from build123d import *

# Parameters (mm, degrees)
F0_R     = 29.1968279335
F1_DEPTH = 46.8261539936
F2_W     = 38.307864219
F2_H     = 7.8112371266
F3_DEPTH = 36.9160473347
F4_R     = 15.8391842582
F5_DEPTH = 29.1978279335
F6_T     = -2.54


with BuildPart() as f1:
    # F0 (on Top) → F1 (new body)
    with BuildSketch(Plane.XY):
        Circle(F0_R)
    extrude(amount=F1_DEPTH)

    # F2 (on face) → F3 (join)
    with BuildSketch(Plane.XY.offset(46.8261539936)):
        with Locations((0, 3.9056185633)):
            Rectangle(F2_W, F2_H)
    extrude(amount=F3_DEPTH)

    # F4 (on face) → F5 (cut, through all)
    with BuildSketch(Plane.XZ):
        with Locations((0, 64.5071235189)):
            Circle(F4_R)
        with BuildLine():
            ThreePointArc((-19.1539321095, 65.2841776609), (0, 83.6768112679), (19.1539321095, 65.2841776609))
            Line((19.1539321095, 65.2841776609), (19.1539321095, 83.7422013283))
            Line((19.1539321095, 83.7422013283), (-19.1539321095, 83.7422013283))
            Line((-19.1539321095, 83.7422013283), (-19.1539321095, 65.2841776609))
        make_face()
    extrude(amount=-F5_DEPTH, mode=Mode.SUBTRACT)

    # F6
    f6_openings = [f1.faces().sort_by_distance(p)[0] for p in [
        (0, 0, 0),
    ]]
    offset(amount=F6_T, openings=f6_openings, kind=Kind.INTERSECTION)


solid = f1.part
Source: CAD feature listing. Evaluate the final solid. Frame: model axes, mm. A direction names the side the tool comes from. Round coordinates to 2 decimals unless told otherwise and drop trailing zeros. Loops run counter-clockwise (first coordinate to the right, second up) from the corner with the lowest first, then second, coordinate; pieces in that order, holes last. Notation, with made-up numbers: (-5, 3.5) -> (0, 3.5) arc R36 cw to (0, 40.5) -> close; hole circle Ø1 at (23, -21.75). An arc over 180 degrees is marked (long way). Answer as a JSON object with one key per item and string values. Group by question number.
Q1. Section query B-B (z = 71.5). Output: boundary loops of the cut face in (x, y).
Q2. Access query for faces 4 (the flat face through (19.154, 4, 56)), 5 (the cylindrical face through (-5.779, -26.023, 21.833)), 6 (the flat face through (-19.154, 4, 56)). Directions: +Z, -Z, +X, -X, +Y, -Y. A direction counts if a zero-diameter tool reaches every point of the face in a straight line with its end or side. Return the directions, or none.
Q3. Mould query, pull axis X, two halves, no side actions, for faces 1 (the cylindrical face through (-0.411, 3.851, 83.672)), 2 (the flat face through (-2.927, 0, 48.787)), 3 (the cylindrical face through (-0.29, 3.89, 46.13)). Classes: pulls with the +X half, pulls with the -X half, needs draft (parallel to the pull), parting line crosses it, or undercut.
Q4. Section query C-C (y = 15). Output: boundary loops of the cut face in (x, z), plus the area to 3 significant figures.
Q5. Section query D-D (x = -21). Output: boundary loops of the cut face in (y, z), plus the area to 3 significant figures.
Q6. Section query A-A (x = 0). Output: boundary loops of the cut face in (y, z), plus the area to 3 significant figures.
Q7. Contact query for flat-ended pins moving along their axis: P1, Ø5, axis at y = 3.5, z = 12, coming from the -X side; P2, Ø4, axis at y = 2.5, z = 59.5, coming from the -X side; P3, Ø5, axis at x = -22, y = 15, coming from the +Z side; P4, Ø11, axis at x = -5, z = 65, coming from the -Y side. Output: stop coordinate, or through.
Q8. Ray query, line 1 (Y direction, x = 0, z = 29); line 2 (X direction, y = -1, z = 6.5); line 3 (Z direction, x = 0, y = 2.25). Return the intervals inside material, ascending. Write a range as from..to.
Completed:
{
 "1": {"outline": "(-17.85, 0) -> (-14.21, 0) -> (-14.21, 7.81) -> (-17.85, 7.81) -> close; (14.21, 0) -> (17.85, 0) -> (17.85, 7.81) -> (14.21, 7.81) -> close"},
 "2": {"face 4": "+Z, +X, +Y, -Y", "face 5": "-Z", "face 6": "+Z, -X, +Y, -Y"},
 "3": {"face 1": "parting line crosses it", "face 2": "needs draft", "face 3": "undercut"},
 "4": {"outline": "(-25.05, 0) -> (-22.04, 0) -> (-22.04, 44.29) -> (22.04, 44.29) -> (22.04, 0) -> (25.05, 0) -> (25.05, 46.83) -> (-25.05, 46.83) -> close", "area": "394 mm²"},
 "5": {"outline": "(-20.28, 0) -> (-16.42, 0) -> (-16.42, 44.29) -> (16.42, 44.29) -> (16.42, 0) -> (20.28, 0) -> (20.28, 46.83) -> (-20.28, 46.83) -> close", "area": "445 mm²"},
 "6": {"outline": "(-29.2, 0) -> (-26.66, 0) -> (-26.66, 44.29) -> (2.54, 44.29) -> (2.54, 46.13) -> (5.27, 46.13) -> (5.27, 44.29) -> (26.66, 44.29) -> (26.66, 0) -> (29.2, 0) -> (29.2, 46.83) -> (7.81, 46.83) -> (7.81, 48.67) -> (0, 48.67) -> (0, 46.83) -> (-29.2, 46.83) -> close; (0, 80.35) -> (7.81, 80.35) -> (7.81, 83.68) -> (0, 83.68) -> close", "area": "409 mm²"},
 "7": {"P1": "x = -29.18", "P2": "x = -19.15", "P3": "z = 46.83", "P4": "through"},
 "8": {"line 1": "-29.2..-26.66, 26.66..29.2", "line 2": "-29.18..-26.64, 26.64..29.18", "line 3": "44.29..48.67, 80.35..83.68"}
}
